Here's how the part is built. I have some questions about the finished solid (model axes, mm). Round coordinates to 2 decimals unless told otherwise and drop trailing zeros. Write each loop counter-clockwise with the first axis right and the second up, starting at its lowest first coordinate (ties: lowest second). Pieces come first, ordered by that corner, then holes. Notation, with made-up numbers: M 72,-30 L 118,-30 A26 cw 118,6 Z; hole C 76,53 d8. An arc over 180 degrees is marked long. Use a Markdown table: item, result. Add a question column.
```python
from build123d import *

# Parameters (mm, degrees)
SKETCH1_W             = 393.7
SKETCH1_H             = 457.2
PLATE_DEPTH           = 12.7
STANDARD_LINEAR_COUNT = 4
STANDARD_LINEAR_PITCH = 127


with BuildPart() as part:
    # Sketch1 → Plate (new body)
    with BuildSketch(Plane.XY):
        with Locations((196.85, 228.6)):
            Rectangle(SKETCH1_W, SKETCH1_H)
    extrude(amount=PLATE_DEPTH)

    # Sketch3 → Hole (revolve, cut)
    with BuildSketch(Plane(origin=(44.45, 38.1, 12.7), x_dir=(0, -1, 0), z_dir=(1, 0, 0))):
        Polygon((0, 0), (0, 29.215464931), (6.35, 25.4), (6.35, 0), align=None)
    hole = revolve(axis=Axis((44.45, 38.1, 19.05), (0, 0, -1)), mode=Mode.SUBTRACT)

    # Standard Linear: Hole ×4
    with Locations(*[(0, i * STANDARD_LINEAR_PITCH, 0) for i in range(1, STANDARD_LINEAR_COUNT)]):
        add(hole, mode=Mode.SUBTRACT)

    # Sketch-Pattern1: Hole at 3 more places
    with Locations((189.2039, 227.04468, 0), (269.22695, 323.07234, 0), (144.04149, 172.849788, 0)):
        add(hole, mode=Mode.SUBTRACT)


solid = part.part
```
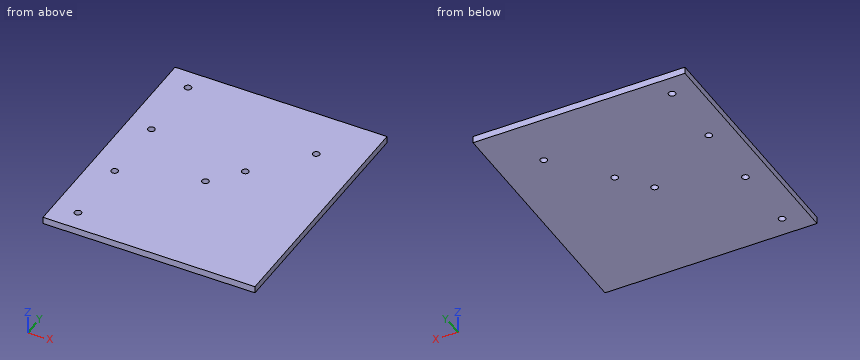
Item 1: I need wall thicknesses on probe 1 along Y at (x, z) = (44.45, 7.75); probe 2 along X at (y, z) = (419.1, 8.75); probe 3 along X at (y, z) = (170.5, 7). Which ranges of each line are inside material? Lowest first, please. Write a range as from..to.
Item 2: Imagine slicing it at B-B on y = 419.1. List the corners of the cut face in (x, z) for me.
Item 3: Imagine slicing it at A-A on x = 44.45. List the corners of the cut face in (y, z) for me.
The answers:
| question | item | result |
|---|---|---|
| 1 | probe 1 | 0..31.75, 44.45..158.75, 171.45..285.75, 298.45..412.75, 425.45..457.2 |
| 1 | probe 2 | 0..38.1, 50.8..393.7 |
| 1 | probe 3 | 0..41.11, 47.79..393.7 |
| 2 | outline | M 0,0 L 38.1,0 L 38.1,12.7 L 0,12.7 Z; M 50.8,0 L 393.7,0 L 393.7,12.7 L 50.8,12.7 Z |
| 3 | outline | M 0,0 L 31.75,0 L 31.75,12.7 L 0,12.7 Z; M 44.45,0 L 158.75,0 L 158.75,12.7 L 44.45,12.7 Z; M 171.45,0 L 285.75,0 L 285.75,12.7 L 171.45,12.7 Z; M 298.45,0 L 412.75,0 L 412.75,12.7 L 298.45,12.7 Z; M 425.45,0 L 457.2,0 L 457.2,12.7 L 425.45,12.7 Z |
